Design review of the part built by this model. Coordinates are the model's own, in mm. A direction names the side the tool comes from. Coordinates: 2 decimals unless noted, no trailing zeros. Loops run counter-clockwise (first coordinate to the right, second up) from the corner with the lowest first, then second, coordinate; pieces in that order, holes last. Notation, with made-up numbers: (25.5, -16.5) -> (68.5, -16.5) arc R16 cw to (68.5, -3.5) -> close; hole circle Ø2 at (-24, -18). An arc over 180 degrees is marked (long way). Use one line per item in the form item = value. Start each with the question number.
1. Consider section D-D (z = 9). State how many separate pieces and enclosed holes the cut face has, then the cut area to 3 significant figures.
2. Machinability: for faces 1 (the face through (21, 1.5, 8)), 2 (the face through (9, 1, 0)), which of the approach directions +Z, -Z, +X, -X, +Y, -Y give a long, thin tool a straight path to every point of the face, cutting with its end or side? Answer none if there is none.
3. For pin 1 (8 mm diameter, centred on x = 30, z = 10, fed in from +Y); pin 2 (8 mm diameter, centred on y = 13, z = 11.5, fed in from +X), all flat-tipped, find the tip position at first contact; note any pin that passes through.
4. Consider section A-A (y = 13.5). State the section outline as (x, z) points, then the cut area to 3 significant figures.
5. Wall thickness on line 1 (X direction, y = 37, z = 8): over which ranges is the line inside the solid? List them lowest first. Write a range as from..to.
6. Consider section C-C (z = 1.5). State the section outline as (x, y) points, then the cut area to 3 significant figures.
from build123d import *

# Parameters (mm, degrees)
BASE_FLANGIA1_DEPTH    = 16
RACCORDO1_R            = 8
RIPETIZIONE_A_L1_COUNT = 2
RIPETIZIONE_A_L1_PITCH = 18.5
RIPETIZIONE_A_L2_COUNT = 2
RIPETIZIONE_A_L2_PITCH = 18.5


# Sheet-metal steps are written as plain solids
with BuildPart() as part:
    # Schizzo1 → Base-Flangia1 (new body)
    with BuildSketch(Plane.XY):
        with BuildLine():
            Line((40, 0), (3, 0))
            ThreePointArc((3, 0), (0.878679656, 0.878679656), (0, 3))
            Line((0, 3), (0, 40))
            Line((0, 40), (1.5, 40))
            Line((1.5, 40), (1.5, 3))
            ThreePointArc((1.5, 3), (1.939339828, 1.939339828), (3, 1.5))
            Line((3, 1.5), (40, 1.5))
            Line((40, 1.5), (40, 0))
        make_face()
    extrude(amount=BASE_FLANGIA1_DEPTH)

    # Raccordo1
    raccordo1_edges = [part.edges().sort_by_distance(p)[0] for p in [
        (40, 0.75, 16),
        (40, 0.75, 0),
        (0.75, 40, 0),
        (0.75, 40, 16),
    ]]
    fillet(raccordo1_edges, radius=RACCORDO1_R - 0.0001)  # a hair under: the kernel refuses the full size

    # Schizzo7 → Foro svasato per Vite M3 a testa svasata (revolve, cut)
    with BuildSketch(Plane(origin=(32, 1.5, 8), x_dir=(0, 0, 1), z_dir=(1, 0, 0))):
        Polygon((0, 0), (0, 1.5), (1.7, 1.5), (1.7, 1.77), (3.47, 0), align=None)
    foro_svasato_per_vite_m3_a_testa_svasata = revolve(axis=Axis((32, 7.85, 8), (0, -1, 0)), mode=Mode.SUBTRACT)

    # Ripetizione a L1: Foro svasato per Vite M3 a testa svasata ×2
    with Locations(*[(-i * RIPETIZIONE_A_L1_PITCH, 0, 0) for i in range(1, RIPETIZIONE_A_L1_COUNT)]):
        add(foro_svasato_per_vite_m3_a_testa_svasata, mode=Mode.SUBTRACT)

    # Schizzo9 → Foro svasato per Vite M3 a testa sva 2 (revolve, cut)
    with BuildSketch(Plane(origin=(1.5, 32, 8), x_dir=(0, 0, -1), z_dir=(0, 1, 0))):
        Polygon((0, 0), (0, 1.5), (1.7, 1.5), (1.7, 1.77), (3.47, 0), align=None)
    foro_svasato_per_vite_m3_a_testa_sva_2 = revolve(axis=Axis((7.85, 32, 8), (-1, 0, 0)), mode=Mode.SUBTRACT)

    # Ripetizione a L2: Foro svasato per Vite M3 a testa sva 2 ×2
    with Locations(*[(0, -i * RIPETIZIONE_A_L2_PITCH, 0) for i in range(1, RIPETIZIONE_A_L2_COUNT)]):
        add(foro_svasato_per_vite_m3_a_testa_sva_2, mode=Mode.SUBTRACT)


solid = part.part
Geometry check:
q1.separate_pieces = 5
q1.enclosed_holes = 0
q1.area = 85.8 mm²
q2.face_1 = +Z, -Z, +X, +Y
q2.face_2 = -Z, +X, -X, +Y, -Y
q3.pin_1 = 1.5
q3.pin_2 = 1.5
q4.outline = (0, 0) -> (1.5, 0) -> (1.5, 4.53) -> (0, 6.03) -> close; (0, 9.97) -> (1.5, 11.47) -> (1.5, 16) -> (0, 16) -> close
q4.area = 15.8 mm²
q5.line_1 = 0..1.5
q6.outline = (0, 3) arc R3 ccw to (3, 0) -> (36.66, 0) -> (36.66, 1.5) -> (3, 1.5) arc R1.5 cw to (1.5, 3) -> (1.5, 36.66) -> (0, 36.66) -> close
q6.area = 106 mm²
